from build123d import *

# Parameters (mm, degrees)
SKETCH1_R           = 5.715
BOSS_EXTRUDE1_DEPTH = 9.968992
SKETCH2_R           = 2.3876
CUT_EXTRUDE1_DEPTH  = 10.968992
SKETCH3_R           = 4
CUT_EXTRUDE2_DEPTH  = 6.35
BOSS_EXTRUDE2_DEPTH = 6.35


with BuildPart() as part:
    # Sketch1 → Boss-Extrude1 (new body)
    with BuildSketch(Plane.XY):
        Circle(SKETCH1_R)
    extrude(amount=BOSS_EXTRUDE1_DEPTH)

    # Sketch2 → Cut-Extrude1 (cut, through all)
    with BuildSketch(Plane(origin=(0, 0, 0), x_dir=(-1, 0, 0), z_dir=(0, 0, -1))):
        Circle(SKETCH2_R)
    extrude(amount=-CUT_EXTRUDE1_DEPTH, mode=Mode.SUBTRACT)

    # Sketch3 → Cut-Extrude2 (cut)
    with BuildSketch(Plane.XY.offset(9.968992)):
        Circle(SKETCH3_R)
    extrude(amount=-CUT_EXTRUDE2_DEPTH, mode=Mode.SUBTRACT)

    # Sketch4 → Boss-Extrude2 (add)
    with BuildSketch(Plane.XY.offset(9.968992)):
        with BuildLine():
            Line((2.54, 3.090048543), (-2.54, 3.090048543))
            ThreePointArc((-2.54, 3.090048543), (0, 4), (2.54, 3.090048543))
        make_face()
    extrude(amount=-BOSS_EXTRUDE2_DEPTH)


solid = part.part
Design review of the part built by this model. Coordinates are the model's own, in mm. A direction names the side the tool comes from. Give positions to 0.01 mm unless a question says otherwise; leave off trailing zeros. Order: outer loops, then holes, each group sorted by start corner. A loop starts at its lowest first (then second) coordinate and runs counter-clockwise, first axis right, second up. Notation, with made-up numbers: (54.25, 85) - (86.25, 85) arc R23 cw to (86.25, 103) - close; hole circle Ø3 at (-15.5, 61). An arc over 180 degrees is marked (long way). Use CSV: the item, a comma, the result in double quotes. Start each with the question number.
Q1. Take a section at A-A (x = 0). State the section outline as (y, z) points (3 decimals).
Q2. For line 1 (Y direction, x = 0, z = 5) (3 decimals); line 2 (Y direction, x = 0, z = 2.55) (3 decimals); line 3 (Z direction, x = 3, y = 1.75), list the stretches that pass through material, from the lowest coordinate up.
Q3. Take a section at C-C (z = 4.5). State the section outline as (x, y) points (3 decimals).
Q4. Take a section at B-B (y = 0). State the section outline as (x, z) points (3 decimals), and give its area (3 significant figures).
Q5. Draft analysis for pull direction Y (two halves, no side actions). For faces 1 (the face through (5.45, 1.72, 4.91)), 2 (the face through (0.52, -2.33, 1.78)), 3 (the face through (0, 4, 9.969)), state which applies: pulls with the +Y half, pulls with the -Y half, needs draft (parallel to the pull), parting line crosses it, or undercut.
Q6. For P1, Ø5, axis at y = 1.5, z = 3, coming from the +X side (3 decimals); P2, Ø3, axis at x = 0, y = 0, coming from the +Z side; P3, Ø2, axis at x = 2.5, z = 3, coming from the -Y side; P4, Ø1, axis at y = 3.5, z = 8.5, coming from the -X side, all flat-tipped, find the tip position at first contact; note any pin that passes through.
Q7. Machinability: for faces 4 (the face through (0, -4, 7)), 5 (the face through (1.2, -2.5, 0)), which of the approach directions +Z, -Z, +X, -X, +Y, -Y give a long, thin tool a straight path to every point of the face, cutting with its end or side? Answer none if there is none.
Q8. Take a section at D-D (x = -3). State the section outline as (y, z) points, and give its area (3 significant figures).
Calculated:
1,outline,"(-5.715, 0) - (-2.388, 0) - (-2.388, 3.619) - (-4, 3.619) - (-4, 9.969) - (-5.715, 9.969) - close; (2.388, 0) - (5.715, 0) - (5.715, 9.969) - (3.09, 9.969) - (3.09, 3.619) - (2.388, 3.619) - close"
2,line 1,"y = -5.715 to -4, 3.09 to 5.715"
2,line 2,"y = -5.715 to -2.388, 2.388 to 5.715"
2,line 3,"z = 0 to 3.62"
3,outline,"circle Ø11.43 at (0, 0); hole (-2.54, 3.09) arc R4 ccw (long way) to (2.54, 3.09) - close"
4,outline,"(-5.715, 0) - (-2.388, 0) - (-2.388, 3.619) - (-4, 3.619) - (-4, 9.969) - (-5.715, 9.969) - close; (2.388, 0) - (5.715, 0) - (5.715, 9.969) - (4, 9.969) - (4, 3.619) - (2.388, 3.619) - close"
4,area,"45.9 mm²"
5,face 1,"parting line crosses it"
5,face 2,"undercut"
5,face 3,"needs draft"
6,P1,"stops at x = 5.715"
6,P2,"passes through"
6,P3,"stops at y = -5.51"
6,P4,"stops at x = -4.86"
7,face 4,"+Z"
7,face 5,"-Z, +X, -X, +Y, -Y"
8,outline,"(-4.86, 0) - (4.86, 0) - (4.86, 9.97) - (2.65, 9.97) - (2.65, 3.62) - (-2.65, 3.62) - (-2.65, 9.97) - (-4.86, 9.97) - close"
8,area,"63.4 mm²"
